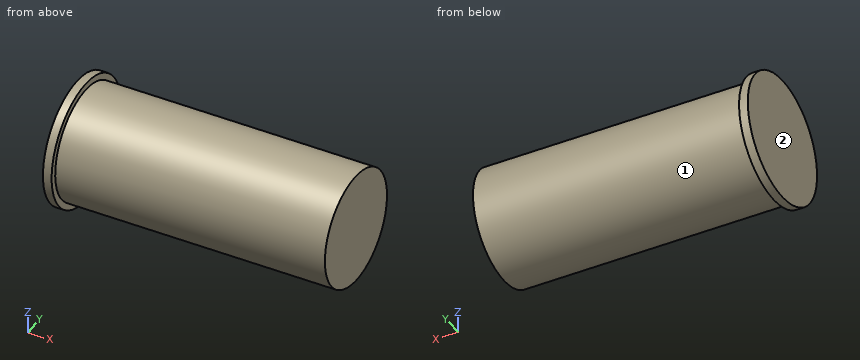
from build123d import *

# Parameters (mm, degrees)
CYLINDER001_R          = 7.25
CYLINDER001_DEPTH      = 1
CYLINDER_R             = 6.5
CYLINDER_DEPTH         = 32
FUSION_PLACEMENT_ANGLE = 90


with BuildPart() as cylinder001:
    # Cylinder001 → Cylinder001 (new body)
    with BuildSketch(Plane.XY):
        Circle(CYLINDER001_R)
    extrude(amount=CYLINDER001_DEPTH)


with BuildPart() as lasermoduletemplate:
    # Cylinder → Cylinder (new body)
    with BuildSketch(Plane.XY):
        Circle(CYLINDER_R)
    extrude(amount=CYLINDER_DEPTH)

    # Fusion: union Cylinder001
    add(cylinder001.part)


with BuildPart() as lasermoduletemplate_1:
    # Fusion placement: moved
    add(lasermoduletemplate.part.moved(Location((-7.5, 0, 7.5))).rotate(Axis((-7.5, 0, 7.5), (0, 1, 0)), FUSION_PLACEMENT_ANGLE))


solid = lasermoduletemplate_1.part
Model file for the job. Use its own axes, mm. Face numbers are marked on the shaded views. A direction names the side the tool comes from. Give positions to 0.01 mm unless a question says otherwise; leave off trailing zeros. Loops run counter-clockwise (first coordinate to the right, second up) from the corner with the lowest first, then second, coordinate; pieces in that order, holes last.
1) Flat gauge pins, fed straight in: pin 1 Ø6 at (x, z) = (7.5, 4) entering from +Y; pin 2 Ø4 at (x, y) = (4, -5) entering from -Z; pin 3 Ø4 at (x, z) = (4.5, 3.5) entering from +Y. Where does each tip first touch, or does it go through?
2) Saw through at B-B (z = 7.5). Write the cut outline in (x, y), plus the area to 4 significant figures.
3) Wall check: line 1 (Z direction, x = -5.5, y = 0.25); line 2 (X direction, y = 5.75, z = 4.25); line 3 (Z direction, x = 13.5, y = -3.25). Give the ranges that are in metal, low to high.
4) Saw through at A-A (y = 0). Write the cut outline in (x, z).
5) Tool access for the marked faces 1 and 2: list every direction of +Z, -Z, +X, -X, +Y, -Y with a clear straight run to the whole face (end or side of a thin tool).
6) Saw through at C-C (x = -1.5). Write the cut outline in (y, z).
Answer block:
1. pin 1: stops at y = 6.48
1. pin 2: stops at z = 1.73
1. pin 3: stops at y = 6.18
2. outline: (-7.5, -7.25) - (-6.5, -7.25) - (-6.5, -6.5) - (24.5, -6.5) - (24.5, 6.5) - (-6.5, 6.5) - (-6.5, 7.25) - (-7.5, 7.25) - close
2. area: 417.5 mm2
3. line 1: z = 1 to 14
3. line 2: x = -7.5 to -6.5
3. line 3: z = 1.87 to 13.13
4. outline: (-7.5, 0.25) - (-6.5, 0.25) - (-6.5, 1) - (24.5, 1) - (24.5, 14) - (-6.5, 14) - (-6.5, 14.75) - (-7.5, 14.75) - close
5. face 1: +X
5. face 2: +Z, -Z, -X, +Y, -Y
6. outline: circle Ø13 at (0, 7.5)
